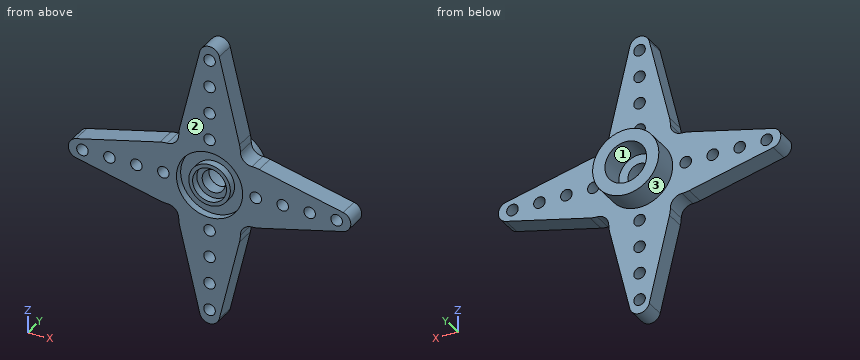
from build123d import *

# Parameters (mm, degrees)
BOSS_EXTRUDE1_DEPTH         = 2.6
SKETCH2_R                   = 1.5
CUT_EXTRUDE1_DEPTH          = 27.066668372
SKETCH3_R                   = 0.75
CUT_EXTRUDE2_DEPTH          = 27.066668372
LPATTERN1_COUNT             = 4
LPATTERN1_PITCH             = 3.5
CIRPATTERN1_COUNT           = 4
CIRPATTERN1_COPY_1_SKETCH_R = 0.75
CIRPATTERN1_COPY_1_DEPTH    = 27.066668372
CIRPATTERN1_COPY_2_SKETCH_R = 0.75
CIRPATTERN1_COPY_2_DEPTH    = 27.066668372
CIRPATTERN1_COPY_3_SKETCH_R = 0.75
CIRPATTERN1_COPY_3_DEPTH    = 27.066668372
CIRPATTERN1_COPY_4_SKETCH_R = 0.75
CIRPATTERN1_COPY_4_DEPTH    = 27.066668372
CIRPATTERN1_COPY_5_SKETCH_R = 0.75
CIRPATTERN1_COPY_5_DEPTH    = 27.066668372
CIRPATTERN1_COPY_6_SKETCH_R = 0.75
CIRPATTERN1_COPY_6_DEPTH    = 27.066668372
CIRPATTERN1_COPY_7_SKETCH_R = 0.75
CIRPATTERN1_COPY_7_DEPTH    = 27.066668372
CIRPATTERN1_COPY_8_SKETCH_R = 0.75
CIRPATTERN1_COPY_8_DEPTH    = 27.066668372
CIRPATTERN1_COPY_9_SKETCH_R = 0.75
CIRPATTERN1_COPY_9_DEPTH    = 27.066668372
SKETCH4_R                   = 4.3
SKETCH4_R_2                 = 2.7
BOSS_EXTRUDE2_DEPTH         = 3.3
SKETCH5_R                   = 4.3
SKETCH5_R_2                 = 2.7
SKETCH5_R_3                 = 2.2
SKETCH5_R_4                 = 1.5
CUT_EXTRUDE3_DEPTH          = 1


with BuildPart() as part:
    # Sketch1 → Boss-Extrude1 (new body)
    with BuildSketch(Plane(origin=(0, 0, 0), x_dir=(1, 0, 0), z_dir=(0, 1, 0))):
        with BuildLine():
            Line((-1.263917336, 17.344159445), (-3.888976418, 6.435875217))
            ThreePointArc((-3.888976418, 6.435875217), (-3.972147132, 5.971218807), (-4, 5.5))
            ThreePointArc((-4, 5.5), (-4.439339828, 4.439339828), (-5.5, 4))
            ThreePointArc((-5.5, 4), (-5.971218807, 3.972147132), (-6.435875217, 3.888976418))
            Line((-6.435875217, 3.888976418), (-17.344159445, 1.263917336))
            ThreePointArc((-17.344159445, 1.263917336), (-18.34, 0), (-17.344159445, -1.263917336))
            Line((-17.344159445, -1.263917336), (-6.435875217, -3.888976418))
            ThreePointArc((-6.435875217, -3.888976418), (-5.971218807, -3.972147132), (-5.5, -4))
            ThreePointArc((-5.5, -4), (-4.439339828, -4.439339828), (-4, -5.5))
            ThreePointArc((-4, -5.5), (-3.972147132, -5.971218807), (-3.888976418, -6.435875217))
            Line((-3.888976418, -6.435875217), (-1.263917336, -17.344159445))
            ThreePointArc((-1.263917336, -17.344159445), (0, -18.34), (1.263917336, -17.344159445))
            Line((1.263917336, -17.344159445), (3.888976418, -6.435875217))
            ThreePointArc((3.888976418, -6.435875217), (3.972147132, -5.971218807), (4, -5.5))
            ThreePointArc((4, -5.5), (4.439339828, -4.439339828), (5.5, -4))
            ThreePointArc((5.5, -4), (5.971218807, -3.972147132), (6.435875217, -3.888976418))
            Line((6.435875217, -3.888976418), (17.344159445, -1.263917336))
            ThreePointArc((17.344159445, -1.263917336), (18.34, 0), (17.344159445, 1.263917336))
            Line((17.344159445, 1.263917336), (6.435875217, 3.888976418))
            ThreePointArc((6.435875217, 3.888976418), (5.971218807, 3.972147132), (5.5, 4))
            ThreePointArc((5.5, 4), (4.439339828, 4.439339828), (4, 5.5))
            ThreePointArc((4, 5.5), (3.972147132, 5.971218807), (3.888976418, 6.435875217))
            Line((3.888976418, 6.435875217), (1.263917336, 17.344159445))
            ThreePointArc((1.263917336, 17.344159445), (0, 18.34), (-1.263917336, 17.344159445))
        make_face()
    extrude(amount=BOSS_EXTRUDE1_DEPTH)

    # Sketch2 → Cut-Extrude1 (cut, through all)
    with BuildSketch(Plane(origin=(0, 2.6, 0), x_dir=(1, 0, 0), z_dir=(0, 1, 0))):
        with Locations(Location((0, 0, 0), (0, 0, 270))):
            Circle(SKETCH2_R)
    extrude(amount=-CUT_EXTRUDE1_DEPTH, mode=Mode.SUBTRACT)

    # Sketch3 → Cut-Extrude2 (cut, through all)
    with BuildSketch(Plane(origin=(0, 2.6, 0), x_dir=(1, 0, 0), z_dir=(0, 1, 0))):
        with Locations(Location((0, 6, 0), (0, 0, 270))):
            Circle(SKETCH3_R)
    cut_extrude2 = extrude(amount=-CUT_EXTRUDE2_DEPTH, mode=Mode.SUBTRACT)

    # LPattern1: Cut-Extrude2 ×4
    with Locations(*[(0, 0, -i * LPATTERN1_PITCH) for i in range(1, LPATTERN1_COUNT)]):
        add(cut_extrude2, mode=Mode.SUBTRACT)

    # CirPattern1: Cut-Extrude2 ×4 about axis
    cirpattern1_axis = Axis((0, 0, 0), (0, 1, 0))
    for i in range(1, CIRPATTERN1_COUNT):
        add(cut_extrude2.rotate(cirpattern1_axis, i * 360 / CIRPATTERN1_COUNT), mode=Mode.SUBTRACT)

    # CirPattern1 copy 1 sketch → CirPattern1 copy 1 (cut, through all)
    with BuildSketch(Plane(origin=(-3.5, 2.6, 0), x_dir=(0, 0, -1), z_dir=(0, 1, 0))):
        with Locations(Location((0, 6, 0), (0, 0, 270))):
            Circle(CIRPATTERN1_COPY_1_SKETCH_R)
    extrude(amount=-CIRPATTERN1_COPY_1_DEPTH, mode=Mode.SUBTRACT)

    # CirPattern1 copy 2 sketch → CirPattern1 copy 2 (cut, through all)
    with BuildSketch(Plane(origin=(0, 2.6, 3.5), x_dir=(-1, 0, 0), z_dir=(0, 1, 0))):
        with Locations(Location((0, 6, 0), (0, 0, 270))):
            Circle(CIRPATTERN1_COPY_2_SKETCH_R)
    extrude(amount=-CIRPATTERN1_COPY_2_DEPTH, mode=Mode.SUBTRACT)

    # CirPattern1 copy 3 sketch → CirPattern1 copy 3 (cut, through all)
    with BuildSketch(Plane(origin=(3.5, 2.6, 0), x_dir=(0, 0, 1), z_dir=(0, 1, 0))):
        with Locations(Location((0, 6, 0), (0, 0, 270))):
            Circle(CIRPATTERN1_COPY_3_SKETCH_R)
    extrude(amount=-CIRPATTERN1_COPY_3_DEPTH, mode=Mode.SUBTRACT)

    # CirPattern1 copy 4 sketch → CirPattern1 copy 4 (cut, through all)
    with BuildSketch(Plane(origin=(-7, 2.6, 0), x_dir=(0, 0, -1), z_dir=(0, 1, 0))):
        with Locations(Location((0, 6, 0), (0, 0, 270))):
            Circle(CIRPATTERN1_COPY_4_SKETCH_R)
    extrude(amount=-CIRPATTERN1_COPY_4_DEPTH, mode=Mode.SUBTRACT)

    # CirPattern1 copy 5 sketch → CirPattern1 copy 5 (cut, through all)
    with BuildSketch(Plane(origin=(0, 2.6, 7), x_dir=(-1, 0, 0), z_dir=(0, 1, 0))):
        with Locations(Location((0, 6, 0), (0, 0, 270))):
            Circle(CIRPATTERN1_COPY_5_SKETCH_R)
    extrude(amount=-CIRPATTERN1_COPY_5_DEPTH, mode=Mode.SUBTRACT)

    # CirPattern1 copy 6 sketch → CirPattern1 copy 6 (cut, through all)
    with BuildSketch(Plane(origin=(7, 2.6, 0), x_dir=(0, 0, 1), z_dir=(0, 1, 0))):
        with Locations(Location((0, 6, 0), (0, 0, 270))):
            Circle(CIRPATTERN1_COPY_6_SKETCH_R)
    extrude(amount=-CIRPATTERN1_COPY_6_DEPTH, mode=Mode.SUBTRACT)

    # CirPattern1 copy 7 sketch → CirPattern1 copy 7 (cut, through all)
    with BuildSketch(Plane(origin=(-10.5, 2.6, 0), x_dir=(0, 0, -1), z_dir=(0, 1, 0))):
        with Locations(Location((0, 6, 0), (0, 0, 270))):
            Circle(CIRPATTERN1_COPY_7_SKETCH_R)
    extrude(amount=-CIRPATTERN1_COPY_7_DEPTH, mode=Mode.SUBTRACT)

    # CirPattern1 copy 8 sketch → CirPattern1 copy 8 (cut, through all)
    with BuildSketch(Plane(origin=(0, 2.6, 10.5), x_dir=(-1, 0, 0), z_dir=(0, 1, 0))):
        with Locations(Location((0, 6, 0), (0, 0, 270))):
            Circle(CIRPATTERN1_COPY_8_SKETCH_R)
    extrude(amount=-CIRPATTERN1_COPY_8_DEPTH, mode=Mode.SUBTRACT)

    # CirPattern1 copy 9 sketch → CirPattern1 copy 9 (cut, through all)
    with BuildSketch(Plane(origin=(10.5, 2.6, 0), x_dir=(0, 0, 1), z_dir=(0, 1, 0))):
        with Locations(Location((0, 6, 0), (0, 0, 270))):
            Circle(CIRPATTERN1_COPY_9_SKETCH_R)
    extrude(amount=-CIRPATTERN1_COPY_9_DEPTH, mode=Mode.SUBTRACT)

    # Sketch4 → Boss-Extrude2 (add)
    with BuildSketch(Plane(origin=(0, 2.6, 0), x_dir=(1, 0, 0), z_dir=(0, 1, 0))):
        with Locations(Location((0, 0, 0), (0, 0, 270))):
            Circle(SKETCH4_R)
        with Locations(Location((0, 0, 0), (0, 0, 270))):
            Circle(SKETCH4_R_2, mode=Mode.SUBTRACT)
    extrude(amount=BOSS_EXTRUDE2_DEPTH)

    # Sketch5 → Cut-Extrude3 (cut)
    # profile 1 of 2: a face of its own
    with BuildSketch(Plane.XZ):
        with Locations(Location((0, 0, 0), (0, 0, 90))):
            Circle(SKETCH5_R)
        with Locations(Location((0, 0, 0), (0, 0, 90))):
            Circle(SKETCH5_R_2, mode=Mode.SUBTRACT)
    # profile 2 of 2: a face of its own
    with BuildSketch(Plane.XZ):
        with Locations(Location((0, 0, 0), (0, 0, 270))):
            Circle(SKETCH5_R_3)
        with Locations(Location((0, 0, 0), (0, 0, 90))):
            Circle(SKETCH5_R_4, mode=Mode.SUBTRACT)
    extrude(amount=-CUT_EXTRUDE3_DEPTH, mode=Mode.SUBTRACT)


solid = part.part
Geometry: final body of the model. Coordinates: model frame, mm. Face numbers are marked on the shaded views. Coordinates: 2 decimals unless noted, no trailing zeros. Loops run counter-clockwise (first coordinate to the right, second up) from the corner with the lowest first, then second, coordinate; pieces in that order, holes last. Notation, with made-up numbers: (-24.75, 0.25) - (14.25, 0.25) arc R30 ccw to (14.25, 30.25) - close; hole circle Ø1 at (49, 6.25). An arc over 180 degrees is marked (long way). One line per question, with ' | ' between items. Start each with the question number.
(1) Cut plane D-D on x = 11.5. Output: boundary loops of the cut face in (y, z).
(2) Draft query along X for the marked faces 1, 2 and 3. Return one class per face: +X half, -X half, draft (parallel to the pull), parting line (faces both ways), or undercut.
(3) Cut plane A-A on x = -13. Output: boundary loops of the cut face in (y, z), and give its area (3 significant figures).
(4) Cut plane B-B on z = -16.5. Output: boundary loops of the cut face in (x, y), and give its area (3 significant figures).
(5) Cut plane C-C on y = 3.7. Output: boundary loops of the cut face in (x, z), and give its area (3 significant figures).
(6) First-contact query: pin 1 (8 mm diameter, centred on x = 6.5, z = 1.5, fed in from -Y); pin 2 (2.5 mm diameter, centred on x = 1, z = 0, fed in from +Y); pin 3 (1.5 mm diameter, centred on x = -1, y = 0.5, fed in from -Z). Flat tips, straight axial feed; report the tip coordinate or a pass-through.
(7) Ray query, L1, parallel to Y at x = 1, z = 8; L2, parallel to X at y = 0.6, z = -16.5; L3, parallel to X at y = 2.05, z = -6. Return the intervals inside material, ascending. Write a range as from..to.
Here are the results:
1) outline: (0, -2.67) - (2.6, -2.67) - (2.6, 2.67) - (0, 2.67) - close
2) face 1: undercut | face 2: draft | face 3: parting line
3) outline: (0, -2.31) - (2.6, -2.31) - (2.6, -0.75) - (0, -0.75) - close; (0, 0.75) - (2.6, 0.75) - (2.6, 2.31) - (0, 2.31) - close | area: 8.11 mm²
4) outline: (-1.47, 0) - (-0.75, 0) - (-0.75, 2.6) - (-1.47, 2.6) - close; (0.75, 0) - (1.47, 0) - (1.47, 2.6) - (0.75, 2.6) - close | area: 3.73 mm²
5) outline: circle Ø8.6 at (0, 0); hole circle Ø5.4 at (0, 0) | area: 35.2 mm²
6) pin 1: y = 0 | pin 2: y = 2.6 | pin 3: z = -18.32
7) L1: 0..2.6 | L2: -1.47..-0.75, 0.75..1.47 | L3: -3.97..-0.75, 0.75..3.97
